Autodesk Inventor part; units mm, degrees
ref_plane "YZ Plane" through (0, 0, 0) normal (1, 0, 0) x (0, 1, 0)
ref_plane "XZ Plane" through (0, 0, 0) normal (0, 1, 0) x (-1, 0, 0)
ref_plane "XY Plane" through (0, 0, 0) normal (0, 0, 1) x (1, 0, 0)
sketch "Skizze1" plane through (0, 0, 0) normal (0, 0, 1) x (1, 0, 0)
  circle A0 centre (0, 0) radius 72
  circle A1 centre (0, 0) radius 101.5
  circle A2 centre (0, 0) radius 86.75
  dimension "d0" = 144
  dimension "d1" = 203
  dimension "d2" = 29.5
  dimension "d3" = 14.75
extrude "Extrusion1" add sketch "Skizze1" along normal blind 10 contours A2
sketch "Skizze2" plane through (0, 0, 10) normal (0, 0, 1) x (1, 0, 0)
  line L0 (-55.2958, -55.2958) -> (55.2958, -55.2958)
  line L1 (55.2958, -55.2958) -> (55.2958, 55.2958)
  line L2 (55.2958, 55.2958) -> (-55.2958, 55.2958)
  line L3 (-55.2958, 55.2958) -> (-55.2958, -55.2958)
  line L4 (-55.2958, -55.2958) -> (55.2958, 55.2958) construction
  line L5 (55.2958, -55.2958) -> (-55.2958, 55.2958) construction
  circle A0 centre (0, 0) radius 78.2 construction
  circle A1 centre (0, 0) radius 72 construction
  circle A2 centre (0, 0) radius 86.75 construction
  dimension "d15" = 156.4
hole "Bohrung1" at (-55.2958, 55.2958, 10) at (55.2958, 55.2958, 10) at (55.2958, -55.2958, 10) at (-55.2958, -55.2958, 10) direction (0, 0, -1) diameter 4.9 end through all countersink diameter 9 countersink angle 90
equation "\"d3\" = 0.5 * d2"
properties part number "Drehkranz" material "ABS-Kunststoff"
Verification items for the finished model (mm, model axes). Round coordinates to 2 decimals unless told otherwise and drop trailing zeros. Write each loop counter-clockwise with the first axis right and the second up, starting at its lowest first coordinate (ties: lowest second). Pieces come first, ordered by that corner, then holes. Notation, with made-up numbers: (69.5, 14) -> (95.5, 14) arc R22 ccw to (95.5, 28) -> close; hole circle Ø5 at (-22, 38). An arc over 180 degrees is marked (long way). Write each question's results on one line, items separated by ' | '.
Q1. Draft check along Y on faces 1 (the face through (-33, 65, 0)), 2 (the face through (-18.806, 84.687, 4.93)), 3 (the face through (53.008, 54.106, 8.078)), 4 (the face through (-9.373, -71.387, 4.93)). Enter one of: released by +Y, released by -Y, zero draft, split by the parting line, or undercut.
Derived:
face 1: zero draft | face 2: split by the parting line | face 3: undercut | face 4: undercut
Q2. Go/stop test with flat-tipped pins: pin 1 Ø4 at (x, y) = (-55.3, 55.3) entering from -Z; pin 2 Ø6 at (x, z) = (-47, 6) entering from +Y; pin 3 Ø3 at (y, z) = (-55, 1) entering from +X. Record where each tip stops, or that it passes through.
Derived:
pin 1: passes through | pin 2: stops at y = 74.76 | pin 3: stops at x = 68.29
Q3. Thickness scan on probe 1 along X at (y, z) = (55.5, 3.5); probe 2 along X at (y, z) = (56, 5.5); probe 3 along X at (y, z) = (22, 1.5). Record the ranges inside material, lowest first.
Derived:
probe 1: x = -66.67 to -57.74, -52.85 to -45.87, 45.87 to 52.85, 57.74 to 66.67 | probe 2: x = -66.25 to -57.64, -52.95 to -45.25, 45.25 to 52.95, 57.64 to 66.25 | probe 3: x = -83.91 to -68.56, 68.56 to 83.91
Q4. Sectioned sample at C-C, the plane z = 4. Record the boundary of the cut face in (x, y), and give its area (3 significant figures).
Derived:
outline: circle Ø173.5 at (0, 0); hole circle Ø144 at (0, 0); hole circle Ø4.9 at (-55.3, -55.3); hole circle Ø4.9 at (-55.3, 55.3); hole circle Ø4.9 at (55.3, -55.3); hole circle Ø4.9 at (55.3, 55.3) | area: 7,280 mm²
Q5. Sectioned sample at A-A, the plane x = 0. Record the boundary of the cut face in (y, z), and give its area (3 significant figures).
Derived:
outline: (-86.75, 0) -> (-72, 0) -> (-72, 10) -> (-86.75, 10) -> close; (72, 0) -> (86.75, 0) -> (86.75, 10) -> (72, 10) -> close | area: 295 mm²
